Can you work these out from the model? Positions are in its coordinate system, mm. A direction names the side the tool comes from. Give positions to 0.01 mm unless a question says otherwise; leave off trailing zeros. Loops run counter-clockwise (first coordinate to the right, second up) from the corner with the lowest first, then second, coordinate; pieces in that order, holes last. Notation, with made-up numbers: (76.25, -21) -> (95.25, -21) arc R34 ccw to (95.25, 16) -> close; hole circle Ø4 at (-31, 52). An arc over 180 degrees is marked (long way). Return JSON: item names as keys, results as strings. Group by question number.
Q1. I need wall thicknesses on line 1 along Y through (x, z) = (-25, -62) (3 decimals); line 2 along X through (y, z) = (16, 11) (3 decimals); line 3 along Z through (x, y) = (76, 40) (3 decimals). Which ranges of each line are inside material? Lowest first, please. Write a range as [from, to].
Q2. Suppose I cut it at D-D, the plane y = 25. Count the separate pieces of the cut face and the enclosed holes in it, and give its area (3 significant figures).
Q3. Thinking about a two-plate mould opening in Z: for faces 4 (the flat face through (-1, 3.175, -1)), 5 (the cylindrical face through (-25.028, 35.642, 61.935)), 6 (the flat face through (-2, 51, 79.375)), which applies, pulls with the +Z half, pulls with the -Z half, needs draft (parallel to the pull), parting line crosses it, or undercut?
Q4. Suppose I cut it at A-A, the plane z = 12.7. Please give me the cut outline in (x, y) (3 decimals).
Q5. Will these pins go through, and if not, where does the flat tip stop? pin 1 (5 mm diameter, centred on x = 98.42, z = -73.75, fed in from +Y) (3 decimals); pin 2 (3 mm diameter, centred on y = 33.5, z = -35.5, fed in from +X); pin 3 (3 mm diameter, centred on x = -74.5, y = 13, fed in from -Z); pin 4 (12 mm diameter, centred on y = 18, z = 50.5, fed in from -X).
Q6. Which directions (+Z, -Z, +X, -X, +Y, -Y) give clear straight access to the entire face, cutting with the end or side of a thin tool? Please do faces 1 (the flat face through (-101.6, 23, 1)), 2 (the flat face through (-1, 23, -63.5)), 3 (the flat face through (-1, 29, -60.325)).
Q7. Suppose I cut it at B-B, the plane x = -25.4. Please give me the cut outline in (y, z) (3 decimals), and give its area (3 significant figures).
Q8. Suppose I cut it at C-C, the plane z = -6. Please give me the cut outline in (x, y) (3 decimals), and give its area (3 significant figures).
```python
from build123d import *

# Parameters (mm, degrees)
SKETCH1_W             = 203.2
SKETCH1_H             = 127
BOSS_EXTRUDE1_DEPTH   = 53.975
SKETCH2_W             = 196.85
SKETCH2_H             = 120.65
CUT_EXTRUDE1_DEPTH    = 50.8
SKETCH4_W             = 234.95
SKETCH4_H             = 158.75
SKETCH4_W_2           = 203.2
SKETCH4_H_2           = 127
BOSS_EXTRUDE2_DEPTH   = 6.35
SKETCH7_W             = 212.4456
SKETCH7_H             = 136.2456
SKETCH7_W_2           = 203.2
SKETCH7_H_2           = 127
CUT_EXTRUDE2_DEPTH    = 2.6416
F_8_32_TAPPED_HOLE1_D = 3.4544
FILLET3_R             = 4.6228
FILLET4_R             = 9.2456
CUT_EXTRUDE5_DEPTH    = 143.875
CUT_EXTRUDE6_REACH    = 221.075
CUT_EXTRUDE7_REACH    = 221.075
SKETCH13_R            = 12.55395
F_6_CLEARANCE_HOLE1_D = 3.7973


with BuildPart() as part:
    # Sketch1 → Boss-Extrude1 (new body)
    with BuildSketch(Plane(origin=(0, 0, 0), x_dir=(1, 0, 0), z_dir=(0, 1, 0))):
        Rectangle(SKETCH1_W, SKETCH1_H)
    extrude(amount=BOSS_EXTRUDE1_DEPTH)

    # Sketch2 → Cut-Extrude1 (cut)
    with BuildSketch(Plane(origin=(0, 53.975, 0), x_dir=(1, 0, 0), z_dir=(0, 1, 0))):
        Rectangle(SKETCH2_W, SKETCH2_H)
    extrude(amount=-CUT_EXTRUDE1_DEPTH, mode=Mode.SUBTRACT)

    # Sketch4 → Boss-Extrude2 (add)
    with BuildSketch(Plane(origin=(0, 53.975, 0), x_dir=(1, 0, 0), z_dir=(0, 1, 0))):
        Rectangle(SKETCH4_W, SKETCH4_H)
        Rectangle(SKETCH4_W_2, SKETCH4_H_2, mode=Mode.SUBTRACT)
    extrude(amount=-BOSS_EXTRUDE2_DEPTH)

    # Sketch7 → Cut-Extrude2 (cut)
    with BuildSketch(Plane(origin=(0, 53.975, 0), x_dir=(1, 0, 0), z_dir=(0, 1, 0))):
        Rectangle(SKETCH7_W, SKETCH7_H)
        Rectangle(SKETCH7_W_2, SKETCH7_H_2, mode=Mode.SUBTRACT)
    extrude(amount=-CUT_EXTRUDE2_DEPTH, mode=Mode.SUBTRACT)

    # #8-32 Tapped Hole1 (through all)
    with Locations(Plane(origin=(0, 53.975, 0), x_dir=(1, 0, 0), z_dir=(0, 1, 0))):
        with Locations((55.92445, 73.7489), (111.8489, 73.7489), (111.8489, 24.582966667), (0, 73.7489), (111.8489, -24.582966667), (111.8489, -73.7489), (55.92445, -73.7489), (0, -73.7489), (-55.92445, -73.7489), (-111.8489, -73.7489), (-111.8489, -24.582966667), (-111.8489, 24.582966667), (-111.8489, 73.7489), (-55.92445, 73.7489)):
            Hole(F_8_32_TAPPED_HOLE1_D / 2)

    # Fillet3
    fillet3_edges = [part.edges().sort_by_distance(p)[0] for p in [
        (-101.6, 52.6542, -63.5),
        (101.6, 52.6542, -63.5),
        (101.6, 52.6542, 63.5),
        (-101.6, 52.6542, 63.5),
    ]]
    fillet(fillet3_edges, radius=FILLET3_R)

    # Fillet4
    fillet4_edges = [part.edges().sort_by_distance(p)[0] for p in [
        (-106.2228, 52.6542, -68.1228),
        (106.2228, 52.6542, -68.1228),
        (106.2228, 52.6542, 68.1228),
        (-106.2228, 52.6542, 68.1228),
    ]]
    fillet(fillet4_edges, radius=FILLET4_R)

    # Sketch10 → Cut-Extrude5 (cut, through all)
    with BuildSketch(Plane.XY.offset(63.5)):
        with BuildLine():
            ThreePointArc((-70.843294161, 16.6624), (-76.2, 35.6489), (-81.556705839, 16.6624))
            Line((-81.556705839, 16.6624), (-70.843294161, 16.6624))
        make_face()
        with BuildLine():
            ThreePointArc((81.556705839, 16.6624), (76.2, 35.6489), (70.843294161, 16.6624))
            Line((70.843294161, 16.6624), (81.556705839, 16.6624))
        make_face()
        with BuildLine():
            ThreePointArc((30.756705839, 16.6624), (25.4, 35.6489), (20.043294161, 16.6624))
            Line((20.043294161, 16.6624), (30.756705839, 16.6624))
        make_face()
        with BuildLine():
            ThreePointArc((-20.043294161, 16.6624), (-25.4, 35.6489), (-30.756705839, 16.6624))
            Line((-30.756705839, 16.6624), (-20.043294161, 16.6624))
        make_face()
    extrude(amount=-CUT_EXTRUDE5_DEPTH, mode=Mode.SUBTRACT)

    # Sketch12 → Cut-Extrude6 (cut, up to next)
    with BuildSketch(Plane(origin=(101.6, 0, 0), x_dir=(0, 0, -1), z_dir=(1, 0, 0)), mode=Mode.PRIVATE) as cut_extrude6_sk1:
        with BuildLine():
            ThreePointArc((-20.043294161, 16.6624), (-25.4, 35.6489), (-30.756705839, 16.6624))
            Line((-30.756705839, 16.6624), (-20.043294161, 16.6624))
        make_face()
    cut_extrude6_tool1 = extrude(cut_extrude6_sk1.sketch, amount=-CUT_EXTRUDE6_REACH, mode=Mode.PRIVATE) & part.part
    add(cut_extrude6_tool1.solids().sort_by_distance((101.6, 25.721198, 25.4))[0], mode=Mode.SUBTRACT)
    # Sketch12 → Cut-Extrude6 (cut, up to next)
    with BuildSketch(Plane(origin=(101.6, 0, 0), x_dir=(0, 0, -1), z_dir=(1, 0, 0)), mode=Mode.PRIVATE) as cut_extrude6_sk2:
        with BuildLine():
            ThreePointArc((30.756705839, 16.6624), (25.4, 35.6489), (20.043294161, 16.6624))
            Line((20.043294161, 16.6624), (30.756705839, 16.6624))
        make_face()
    cut_extrude6_tool2 = extrude(cut_extrude6_sk2.sketch, amount=-CUT_EXTRUDE6_REACH, mode=Mode.PRIVATE) & part.part
    add(cut_extrude6_tool2.solids().sort_by_distance((101.6, 25.721198, -25.4))[0], mode=Mode.SUBTRACT)

    # Sketch13 → Cut-Extrude7 (cut, up to next)
    with BuildSketch(Plane.ZY.offset(101.6), mode=Mode.PRIVATE) as cut_extrude7_sk1:
        with Locations((12.7, 28.575)):
            Circle(SKETCH13_R)
    cut_extrude7_tool1 = extrude(cut_extrude7_sk1.sketch, amount=-CUT_EXTRUDE7_REACH, mode=Mode.PRIVATE) & part.part
    add(cut_extrude7_tool1.solids().sort_by_distance((-101.6, 28.575, 12.7))[0], mode=Mode.SUBTRACT)

    # #6 Clearance Hole1 (through all)
    with Locations(Plane(origin=(0, 47.625, 0), x_dir=(-1, 0, 0), z_dir=(0, -1, 0))):
        with Locations((-98.425, 73.7489), (-98.425, -73.7489), (98.425, -73.7489), (98.425, 73.7489)):
            Hole(F_6_CLEARANCE_HOLE1_D / 2)


solid = part.part
```
Ans:
{
 "1": {"line 1": "y = [0, 16.662], [35.641, 53.975]", "line 2": "x = [-101.6, -98.425], [98.425, 101.6]", "line 3": "z = [-63.5, -60.325], [60.325, 63.5]"},
 "2": {"separate pieces": "11", "enclosed holes": "0", "area": "1,330 mm^2"},
 "3": {"face 4": "undercut", "face 5": "needs draft", "face 6": "pulls with the +Z half"},
 "4": {"outline": "(-117.475, 47.625) -> (-101.6, 47.625) -> (-101.6, 41.129) -> (-98.425, 41.129) -> (-98.425, 53.975) -> (-101.6, 53.975) -> (-101.6, 51.333) -> (-106.223, 51.333) -> (-106.223, 53.975) -> (-117.475, 53.975) -> close; (-101.6, 0) -> (101.6, 0) -> (101.6, 47.625) -> (117.475, 47.625) -> (117.475, 53.975) -> (106.223, 53.975) -> (106.223, 51.333) -> (101.6, 51.333) -> (101.6, 53.975) -> (98.425, 53.975) -> (98.425, 3.175) -> (-98.425, 3.175) -> (-98.425, 16.021) -> (-101.6, 16.021) -> close"},
 "5": {"pin 1": "stops at y = 53.975", "pin 2": "stops at x = 101.6", "pin 3": "stops at z = -63.5", "pin 4": "stops at x = -101.6"},
 "6": {"face 1": "+Z, -Z, -X, -Y", "face 2": "-Z, +X, -X, -Y", "face 3": "+Y"},
 "7": {"outline": "(0, -63.5) -> (16.662, -63.5) -> (16.662, -60.325) -> (3.175, -60.325) -> (3.175, 60.325) -> (16.662, 60.325) -> (16.662, 63.5) -> (0, 63.5) -> close; (35.649, -63.5) -> (47.625, -63.5) -> (47.625, -79.375) -> (53.975, -79.375) -> (53.975, -68.123) -> (51.333, -68.123) -> (51.333, -63.5) -> (53.975, -63.5) -> (53.975, -60.325) -> (35.649, -60.325) -> close; (35.649, 60.325) -> (53.975, 60.325) -> (53.975, 63.5) -> (51.333, 63.5) -> (51.333, 68.123) -> (53.975, 68.123) -> (53.975, 79.375) -> (47.625, 79.375) -> (47.625, 63.5) -> (35.649, 63.5) -> close", "area": "782 mm^2"},
 "8": {"outline": "(-117.475, 47.625) -> (-101.6, 47.625) -> (-101.6, 0) -> (101.6, 0) -> (101.6, 47.625) -> (117.475, 47.625) -> (117.475, 53.975) -> (106.223, 53.975) -> (106.223, 51.333) -> (101.6, 51.333) -> (101.6, 53.975) -> (98.425, 53.975) -> (98.425, 3.175) -> (-98.425, 3.175) -> (-98.425, 53.975) -> (-101.6, 53.975) -> (-101.6, 51.333) -> (-106.223, 51.333) -> (-106.223, 53.975) -> (-117.475, 53.975) -> close", "area": "1,140 mm^2"}
}
